from build123d import *

# Parameters (mm, degrees)
ESQUISSE1_W             = 70
ESQUISSE1_H             = 110
BOSS_EXTRU_1_DEPTH      = 6
ENL_V_MAT_EXTRU_1_DEPTH = 131.522028792
ESQUISSE3_R             = 1.5
ENL_V_MAT_EXTRU_2_DEPTH = 131.522028792
ESQUISSE4_R             = 2.995
ENL_V_MAT_EXTRU_3_DEPTH = 3


with BuildPart() as part:
    # Esquisse1 → Boss.-Extru.1 (new body)
    with BuildSketch(Plane.XY):
        with Locations((-35, 55)):
            Rectangle(ESQUISSE1_W, ESQUISSE1_H)
    extrude(amount=BOSS_EXTRU_1_DEPTH)

    # Esquisse2 → Enlèv. mat.-Extru.1 (cut, through all)
    with BuildSketch(Plane(origin=(0, 0, 0), x_dir=(-1, 0, 0), z_dir=(0, 0, -1))):
        Polygon((0, 110), (25, 110), (25, 104), (6, 104), (6, 68.5), (0, 68.5), align=None)
        Polygon((70, 110), (45, 110), (45, 104), (64, 104), (64, 68.5), (70, 68.5), align=None)
        Polygon((0, 0), (25, 0), (25, 6), (6, 6), (6, 38.5), (0, 38.5), align=None)
        Polygon((45, 0), (70, 0), (70, 38.5), (64, 38.5), (64, 6), (45, 6), align=None)
    extrude(amount=-ENL_V_MAT_EXTRU_1_DEPTH, mode=Mode.SUBTRACT)

    # Esquisse3 → Enlèv. mat.-Extru.2 (cut, through all)
    with BuildSketch(Plane(origin=(0, 0, 0), x_dir=(-1, 0, 0), z_dir=(0, 0, -1))):
        with Locations((3, 53.5)):
            Circle(ESQUISSE3_R)
    extrude(amount=-ENL_V_MAT_EXTRU_2_DEPTH, mode=Mode.SUBTRACT)

    # Esquisse4 → Enlèv. mat.-Extru.3 (cut)
    with BuildSketch(Plane(origin=(0, 0, 0), x_dir=(-1, 0, 0), z_dir=(0, 0, -1))):
        with Locations((3, 53.5)):
            Circle(ESQUISSE4_R)
    extrude(amount=-ENL_V_MAT_EXTRU_3_DEPTH, mode=Mode.SUBTRACT)


solid = part.part
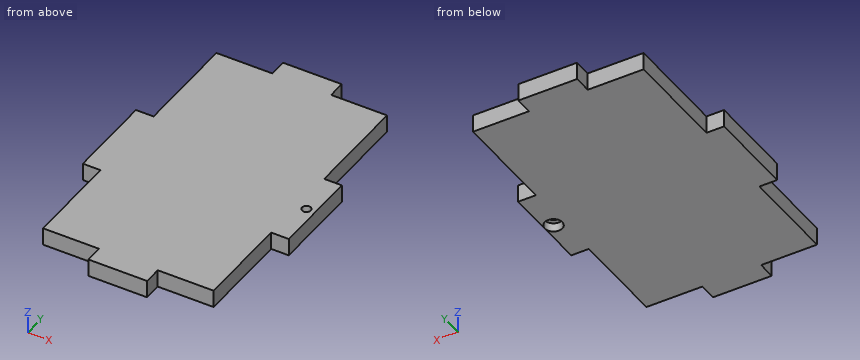
Design review of the part built by this model. Coordinates are the model's own, in mm. Give positions to 0.01 mm unless a question says otherwise; leave off trailing zeros. Write each loop counter-clockwise with the first axis right and the second up, starting at its lowest first coordinate (ties: lowest second). Pieces come first, ordered by that corner, then holes. Notation, with made-up numbers: M 86,43.5 L 144,43.5 A22 cw 144,50.5 Z; hole C 8.25,84 d2. An arc over 180 degrees is marked long. Answer as a JSON object with one key per item and string values. Group by question number.
1) Clearance check with flat-ended pins moving along their axes: pin 1 Ø1.8 at (x, z) = (-68, 2) entering from +Y; pin 2 Ø1.8 at (x, z) = (-56, 1.5) entering from -Y; pin 3 Ø1.8 at (x, z) = (-67.5, 2) entering from -Y. State where each tip first meets the part, or that it passes through.
2) We need section A-A (y = 53.5). Give the boundary of the cut face in (x, z) (3 decimals), and give its area (3 significant figures).
3) We need section C-C (x = -3). Give the boundary of the cut face in (y, z) (3 decimals), and give its area (3 significant figures).
4) We need section B-B (z = 4.75). Give the boundary of the cut face in (x, y).
5) For line 1 along Y through (x, z) = (-3, 0.85) (3 decimals); line 2 along X through (y, z) = (73, 3.8); line 3 along Y through (x, z) = (-3, 3.7), list the stretches that pass through material, from the lowest coordinate up.
6) We need section D-D (y = 79). Give the boundary of the cut face in (x, z), and give its area (3 significant figures).
Answer key:
{
 "1": {"pin 1": "stops at y = 68.5", "pin 2": "stops at y = 6", "pin 3": "stops at y = 38.5"},
 "2": {"outline": "M -70,0 L -5.995,0 L -5.995,3 L -4.5,3 L -4.5,6 L -70,6 Z; M -1.5,3 L -0.005,3 L -0.005,0 L 0,0 L 0,6 L -1.5,6 Z", "area": "393 mm²"},
 "3": {"outline": "M 38.5,0 L 50.505,0 L 50.505,3 L 52,3 L 52,6 L 38.5,6 Z; M 55,3 L 56.495,3 L 56.495,0 L 68.5,0 L 68.5,6 L 55,6 Z", "area": "153 mm²"},
 "4": {"outline": "M -70,38.5 L -64,38.5 L -64,6 L -45,6 L -45,0 L -25,0 L -25,6 L -6,6 L -6,38.5 L 0,38.5 L 0,68.5 L -6,68.5 L -6,104 L -25,104 L -25,110 L -45,110 L -45,104 L -64,104 L -64,68.5 L -70,68.5 Z; hole C -3,53.5 d3"},
 "5": {"line 1": "y = 38.5 to 50.505, 56.495 to 68.5", "line 2": "x = -64 to -6", "line 3": "y = 38.5 to 52, 55 to 68.5"},
 "6": {"outline": "M -64,0 L -6,0 L -6,6 L -64,6 Z", "area": "348 mm²"}
}
